```python
from build123d import *

# Parameters (mm, degrees)
SKETCH1_R           = 1
BOSS_EXTRUDE1_DEPTH = 1.5


with BuildPart() as part:
    # Sketch1 → Boss-Extrude1 (new body)
    with BuildSketch(Plane(origin=(0, 0, 0), x_dir=(1, 0, 0), z_dir=(0, 1, 0))):
        with BuildLine():
            Line((0, 0), (28, 0))
            Line((28, 0), (28, 3.880202712))
            ThreePointArc((28, 3.880202712), (24.35, 6.1), (28, 8.319797288))
            Line((28, 8.319797288), (28, 12))
            ThreePointArc((28, 12), (26.607680962, 15.033150178), (23.4, 15.954743987))
            ThreePointArc((23.4, 15.954743987), (14, 22.198039027), (4.6, 15.954743987))
            ThreePointArc((4.6, 15.954743987), (1.392319038, 15.033150178), (0, 12))
            Line((0, 12), (0, 8.319797288))
            ThreePointArc((0, 8.319797288), (3.65, 6.1), (0, 3.880202712))
            Line((0, 3.880202712), (0, 0))
        make_face()
        with Locations((5.9, 12)):
            Circle(SKETCH1_R, mode=Mode.SUBTRACT)
        with Locations((22.1, 12)):
            Circle(SKETCH1_R, mode=Mode.SUBTRACT)
    extrude(amount=BOSS_EXTRUDE1_DEPTH)


solid = part.part
```
Geometry: final body of the model. Coordinates: model frame, mm. Give positions to 0.01 mm unless a question says otherwise; leave off trailing zeros. Loops run counter-clockwise (first coordinate to the right, second up) from the corner with the lowest first, then second, coordinate; pieces in that order, holes last. Notation, with made-up numbers: (-14, -36.5) - (35, -36.5) arc R18 ccw to (35, -13.5) - close; hole circle Ø1 at (20, 17.25). An arc over 180 degrees is marked (long way). Answer as CSV lines item,"result". Start each with the question number.
(1) Section query D-D (z = -15.5). Output: boundary loops of the cut face in (x, y), and give its area (3 significant figures).
(2) Ray query, line 1 along X through (y, z) = (0.3, -12); line 2 along X through (y, z) = (0.5, -12.75); line 3 along Z through (x, y) = (4, 0.7). Return the intervals inside material, ascending. Write a range as [from, to].
(3) Mould query, pull axis Z, two halves, no side actions, for faces 1 (the face through (0, 1, -10)), 2 (the face through (21.1, 0.7, -12)), 3 (the face through (1.429, 0.74, -15.064)). Classes: +Z half, -Z half, draft (parallel to the pull), parting line (faces both ways), or undercut.
(4) Section query B-B (x = 22.5). Output: boundary loops of the cut face in (y, z), and give its area (3 significant figures).
(5) Section query C-C (x = 6). Output: boundary loops of the cut face in (y, z).
(6) Section query A-A (y = 1.05). Output: boundary loops of the cut face in (x, z), and give its area (3 significant figures).
Worked answers:
1,outline,"(2.06, 0) - (25.94, 0) - (25.94, 1.5) - (2.06, 1.5) - close"
1,area,"35.8 mm^2"
2,line 1,"x = [0, 4.9], [6.9, 21.1], [23.1, 28]"
2,line 2,"x = [0.07, 5.24], [6.56, 21.44], [22.76, 27.93]"
2,line 3,"z = [-16, 0]"
3,face 1,"draft"
3,face 2,"undercut"
3,face 3,"-Z half"
4,outline,"(0, -17.63) - (1.5, -17.63) - (1.5, -12.92) - (0, -12.92) - close; (0, -11.08) - (1.5, -11.08) - (1.5, 0) - (0, 0) - close"
4,area,"23.7 mm^2"
5,outline,"(0, -18.32) - (1.5, -18.32) - (1.5, -12.99) - (0, -12.99) - close; (0, -11.01) - (1.5, -11.01) - (1.5, 0) - (0, 0) - close"
6,outline,"(0, -12) arc R4 ccw to (4.6, -15.95) arc R10.2 ccw to (23.4, -15.95) arc R4 ccw to (28, -12) - (28, -8.32) arc R2.5 cw (long way) to (28, -3.88) - (28, 0) - (0, 0) - (0, -3.88) arc R2.5 cw (long way) to (0, -8.32) - close; hole circle Ø2 at (5.9, -12); hole circle Ø2 at (22.1, -12)"
6,area,"488 mm^2"
